Geometry: final body of the model. Coordinates: model frame, mm. A direction names the side the tool comes from. Round coordinates to 2 decimals unless told otherwise and drop trailing zeros. Order: outer loops, then holes, each group sorted by start corner. A loop starts at its lowest first (then second) coordinate and runs counter-clockwise, first axis right, second up. Notation, with made-up numbers: M 7.25,74.25 L 32.25,74.25 A8 ccw 32.25,84.25 Z; hole C 83,63.25 d4. An arc over 180 degrees is marked long. Put each result on its own line as item: value. Start each with the question number.
1) Section A-A, the plane x = -53. Return loops of the section in (y, z), then the cut area to 3 significant figures.
2) First-contact query: P1, Ø14, axis at x = -145.5, y = 16.5, coming from the +Z side; P2, Ø3, axis at y = 36, z = 107.5, coming from the +X side; P3, Ø6.5, axis at x = 18.5, z = -102.5, coming from the -Y side; P4, Ø1.5, axis at x = -15.5, z = 8, coming from the -Y side. Flat tips, straight axial feed; report the tip coordinate or a pass-through.
3) Material intervals for probe 1 along X at (y, z) = (52.65, 72.5); probe 2 along Z at (x, y) = (-166.5, 33); probe 3 along Y at (x, z) = (-43, 93), sorted ascending. Write a range as [from, to].
4) Access query for faces 5 (the flat face through (-168, 27, -108.5)), 6 (the flat face through (-168, 27, 104.5)), 7 (the flat face through (28, 52, 2)). Directions: +Z, -Z, +X, -X, +Y, -Y. A direction counts if a zero-diameter tool reaches every point of the face in a straight line with its end or side. Return the directions, or none.
5) Draft query along X for faces 1 (the flat face through (0, 28, 2)), 2 (the flat face through (-112, 0, 2)), 3 (the flat face through (-217, 3.6, -24.6)), 4 (the cylindrical face through (-119.85, 46.99, 106.47)). Return one class per face: pulls with the +X half, pulls with the -X half, needs draft (parallel to the pull), parting line crosses it, or undercut.
6) Section C-C, the plane z = 91.5. Return loops of the section in (x, y).
7) Section B-B, the plane y = 31. Return loops of the section in (x, z).
8) Section D-D, the plane x = -163. Return loops of the section in (y, z), then the cut area to 3 significant figures.
from build123d import *

# Parameters (mm, degrees)
SM_BASE_FLANGE_1_DEPTH      = 110
HOLE_WIZARD_1_D             = 5.5
HOLE_WIZARD_1_CSINK_D       = 10.6
HOLE_WIZARD_1_CSINK_ANGLE   = 90
HOLE_WIZARD_M3_1_D          = 2.5
CUT_EXTRUDE_2_REACH         = 250.783
SKETCH_19_R                 = 15
FILLET_1_R                  = 5
SKETCH_20_W                 = 100
SKETCH_20_H                 = 1.5
CUT_EXTRUDE_3_DEPTH         = 10
SM_START                    = -217
SM_EDGE_FLANGE_2_DEPTH      = 102
SM_START_2                  = -117
SM_EDGE_FLANGE_2_2_DEPTH    = 2
SM_EDGE_FLANGE_2_3_DEPTH    = 100
HOLE_START                  = -108.5
HOLE_WIZARD_8_2_8_2_1_DEPTH = 4
FILLET_2_R                  = 10


# Read off the part's stored shape, not the designer's step: 边线-法兰2, Ø8.2 (8.2) 直径槽口1
# Sheet-metal steps are written as plain solids
with BuildPart() as part:
    # Sketch1 → 基体-法兰1 (new, symmetric)
    with BuildSketch(Plane.XY):
        with BuildLine():
            Line((-217, 0), (-4.1, 0))
            ThreePointArc((-4.1, 0), (-1.200862197, 1.200862197), (0, 4.1))
            Line((0, 4.1), (0, 51.9))
            ThreePointArc((0, 51.9), (0.029289322, 51.970710678), (0.1, 52))
            Line((0.1, 52), (57, 52))
            Line((57, 52), (57, 56))
            Line((57, 56), (0.1, 56))
            ThreePointArc((0.1, 56), (-2.799137803, 54.799137803), (-4, 51.9))
            Line((-4, 51.9), (-4, 4.1))
            ThreePointArc((-4, 4.1), (-4.029289322, 4.029289322), (-4.1, 4))
            Line((-4.1, 4), (-217, 4))
            Line((-217, 4), (-217, 0))
        make_face()
    extrude(amount=SM_BASE_FLANGE_1_DEPTH, both=True)

    # 打孔尺寸开槽半沉头螺钉的类型1 (through all)
    with Locations(Plane(origin=(0, 56, 0), x_dir=(1, 0, 0), z_dir=(0, 1, 0))):
        with Locations((18.5, -102.5), (18.5, -72.5), (50.5, -72.5), (50.5, -102.5)):
            hole_wizard_1 = CounterSinkHole(HOLE_WIZARD_1_D / 2, HOLE_WIZARD_1_CSINK_D / 2, counter_sink_angle=HOLE_WIZARD_1_CSINK_ANGLE)

    # 镜向2: 打孔尺寸开槽半沉头螺钉的类型1 across plane
    add(hole_wizard_1.mirror(Plane.XY), mode=Mode.SUBTRACT)

    # M3 螺纹孔1 (through all)
    with Locations(Plane(origin=(0, 4, 0), x_dir=(1, 0, 0), z_dir=(0, 1, 0))):
        with Locations((-15.5, 8), (-15.5, -8)):
            Hole(HOLE_WIZARD_M3_1_D / 2)

    # 草图19 → 切除-拉伸2 (cut, up to next)
    with BuildSketch(Plane(origin=(0, 4, 0), x_dir=(1, 0, 0), z_dir=(0, 1, 0)), mode=Mode.PRIVATE) as cut_extrude_2_sk1:
        with Locations(Location((-53, 0, 0), (0, 0, 270))):
            Circle(SKETCH_19_R)
    cut_extrude_2_tool1 = extrude(cut_extrude_2_sk1.sketch, amount=-CUT_EXTRUDE_2_REACH, mode=Mode.PRIVATE) & part.part
    add(cut_extrude_2_tool1.solids().sort_by_distance((-53, 4, 0))[0], mode=Mode.SUBTRACT)

    # 圆角1
    fillet_1_edges = [part.edges().sort_by_distance(p)[0] for p in [
        (57, 54, 110),
        (57, 54, -110),
    ]]
    fillet(fillet_1_edges, radius=FILLET_1_R)

    # 草图20 → 切除-拉伸3 (cut)
    with BuildSketch(Plane(origin=(0, 4, 0), x_dir=(1, 0, 0), z_dir=(0, 1, 0))):
        with Locations((-167, 109.25)):
            Rectangle(SKETCH_20_W, SKETCH_20_H)
    cut_extrude_3 = extrude(amount=-CUT_EXTRUDE_3_DEPTH, mode=Mode.SUBTRACT)

    # 镜向5: 切除-拉伸3 across plane
    add(cut_extrude_3.mirror(Plane.XY), mode=Mode.SUBTRACT)

    # 边线-法兰2 outline → 边线-法兰2 (cut)
    with BuildSketch(Plane.YZ.offset(SM_START)):
        with BuildLine():
            ThreePointArc((4, -108.498780306), (1.16571985, -107.263564213), (0, -104.4))
            Line((0, -104.4), (0, -108.5))
            Line((0, -108.5), (4, -108.5))
            Line((4, -108.5), (4, -108.498780306))
        make_face()
    sm_edge_flange_2 = extrude(amount=SM_EDGE_FLANGE_2_DEPTH, mode=Mode.SUBTRACT)

    # Sm Edge Flange 2 2 outline → Sm Edge Flange 2 2 (cut)
    with BuildSketch(Plane.YZ.offset(SM_START_2)):
        with BuildLine():
            Line((4, -102.4), (0, -102.4))
            Line((0, -102.4), (0, -104.4))
            ThreePointArc((0, -104.4), (1.16571985, -107.263564213), (4, -108.498780306))
            Line((4, -108.498780306), (4, -102.4))
        make_face()
    sm_edge_flange_2_2 = extrude(amount=SM_EDGE_FLANGE_2_2_DEPTH, mode=Mode.SUBTRACT)

    # Sm Edge Flange 2 3 outline → Sm Edge Flange 2 3 (add)
    with BuildSketch(Plane.YZ.offset(SM_START)):
        with BuildLine():
            ThreePointArc((4.1, -104.5), (4.029289322, -104.470710678), (4, -104.4))
            Line((4, -104.4), (4, -108.498780306))
            ThreePointArc((4, -108.498780306), (4.049996281, -108.499695065), (4.1, -108.5))
            Line((4.1, -108.5), (50, -108.5))
            Line((50, -108.5), (50, -104.5))
            Line((50, -104.5), (4.1, -104.5))
        make_face()
    sm_edge_flange_2_3 = extrude(amount=SM_EDGE_FLANGE_2_3_DEPTH)

    # Ø8.2 (8.2) 直径槽口1 outline → Ø8.2 (8.2) 直径槽口1 (cut)
    with BuildSketch(Plane.XY.offset(HOLE_START)):
        with BuildLine():
            ThreePointArc((-202.9, 39.9), (-207, 44), (-211.1, 39.9))
            Line((-211.1, 39.9), (-211.1, 28.1))
            ThreePointArc((-211.1, 28.1), (-207, 24), (-202.9, 28.1))
            Line((-202.9, 28.1), (-202.9, 39.9))
        make_face()
        with BuildLine():
            ThreePointArc((-122.9, 39.9), (-127, 44), (-131.1, 39.9))
            Line((-131.1, 39.9), (-131.1, 28.1))
            ThreePointArc((-131.1, 28.1), (-127, 24), (-122.9, 28.1))
            Line((-122.9, 28.1), (-122.9, 39.9))
        make_face()
    hole_wizard_8_2_8_2_1 = extrude(amount=HOLE_WIZARD_8_2_8_2_1_DEPTH, mode=Mode.SUBTRACT)

    # 镜向6: 边线-法兰2, Sm Edge Flange 2 2, Sm Edge Flange 2 3, Ø8.2 (8.2) 直径槽口1 across plane
    add(sm_edge_flange_2.mirror(Plane.XY), mode=Mode.SUBTRACT)
    add(sm_edge_flange_2_2.mirror(Plane.XY), mode=Mode.SUBTRACT)
    add(sm_edge_flange_2_3.mirror(Plane.XY))
    add(hole_wizard_8_2_8_2_1.mirror(Plane.XY), mode=Mode.SUBTRACT)

    # 圆角2
    fillet_2_edges = [part.edges().sort_by_distance(p)[0] for p in [
        (-117, 50, -106.5),
        (-217, 50, -106.5),
        (-217, 50, 106.5),
        (-117, 50, 106.5),
    ]]
    fillet(fillet_2_edges, radius=FILLET_2_R)


solid = part.part
Result sheet:
1. outline: M 0,-110 L 4,-110 L 4,-15 L 0,-15 Z; M 0,15 L 4,15 L 4,110 L 0,110 Z
1. area: 760 mm2
2. P1: stops at z = 108.5
2. P2: stops at x = 0
2. P3: stops at y = 52
2. P4: passes through
3. probe 1: x = [-3.93, 15.75], [21.25, 47.75], [53.25, 57]
3. probe 2: z = [-108.5, -104.5], [104.5, 108.5]
3. probe 3: y = [0, 4]
4. face 5: -Z, -X, +Y, -Y
4. face 6: -X, +Y
4. face 7: +Z, -Z, +X, -Y
5. face 1: pulls with the +X half
5. face 2: needs draft
5. face 3: pulls with the -X half
5. face 4: undercut
6. outline: M -217,0 L -4.1,0 A4.1 ccw 0,4.1 L 0,51.9 A0.1 cw 0.1,52 L 57,52 L 57,56 L 0.1,56 A4.1 ccw -4,51.9 L -4,4.1 A0.1 cw -4.1,4 L -217,4 Z
7. outline: M -217,-108.5 L -211.1,-108.5 L -211.1,-104.5 L -217,-104.5 Z; M -217,104.5 L -211.1,104.5 L -211.1,108.5 L -217,108.5 Z; M -202.9,-108.5 L -131.1,-108.5 L -131.1,-104.5 L -202.9,-104.5 Z; M -202.9,104.5 L -131.1,104.5 L -131.1,108.5 L -202.9,108.5 Z; M -122.9,-108.5 L -117,-108.5 L -117,-104.5 L -122.9,-104.5 Z; M -122.9,104.5 L -117,104.5 L -117,108.5 L -122.9,108.5 Z; M -4,-110 L 0,-110 L 0,110 L -4,110 Z
8. outline: M 0,-104.4 A4.1 ccw 4.1,-108.5 L 50,-108.5 L 50,-104.5 L 4.1,-104.5 A0.1 cw 4,-104.4 L 4,104.4 A0.1 cw 4.1,104.5 L 50,104.5 L 50,108.5 L 4.1,108.5 A4.1 ccw 0,104.4 Z
8. area: 1,230 mm2
